from build123d import *

# Parameters (mm, degrees)
CUT_EXTRUDE1_DEPTH      = 10
CUT_EXTRUDE1_DEPTH_BACK = 10


with BuildPart() as part:
    # Sketch1 → Revolve1 (revolve)
    with BuildSketch(Plane(origin=(0, 0, 0), x_dir=(0, 0, -1), z_dir=(1, 0, 0))):
        Polygon((-25.1, 0), (-25.1, 5.717157288), (-24.817157288, 6), (205.333333333, 6), (205.333333333, 16), (216, 16), (216, 0), align=None)
    revolve(axis=Axis((0, 0, -216), (0, 0, 1)))

    # Sketch2 → Cut-Extrude1 (cut, two sides)
    with BuildSketch(Plane(origin=(0, 0, 0), x_dir=(1, 0, 0), z_dir=(0, 1, 0))) as cut_extrude1_sk:
        Polygon((-10, -39.1), (10, -39.1), (10, -19.1), (5, -19.1), (5, -31.1), (-5, -31.1), (-5, -19.1), (-10, -19.1), align=None)
    extrude(amount=CUT_EXTRUDE1_DEPTH, mode=Mode.SUBTRACT)
    extrude(cut_extrude1_sk.sketch, amount=-CUT_EXTRUDE1_DEPTH_BACK, mode=Mode.SUBTRACT)

    # Sketch3 → Revolve2 (revolve)
    with BuildSketch(Plane(origin=(0, 0, 0), x_dir=(0, 0, -1), z_dir=(1, 0, 0))):
        with BuildLine():
            Line((-47.1, 0), (-47.1, 4.233))
            Line((-47.1, 4.233), (-46.333, 5))
            Line((-46.333, 5), (-29.072729678, 5))
            Line((-29.072729678, 5), (-26.699415898, 4.136184428))
            ThreePointArc((-26.699415898, 4.136184428), (-26.598392718, 4.109115348), (-26.494203812, 4.1))
            Line((-26.494203812, 4.1), (-25.7, 4.1))
            ThreePointArc((-25.7, 4.1), (-25.275735931, 4.275735931), (-25.1, 4.7))
            Line((-25.1, 4.7), (-24.5, 4.7))
            Line((-24.5, 4.7), (-24.5, 0))
            Line((-24.5, 0), (-47.1, 0))
        make_face()
    revolve(axis=Axis((0, 0, 24.5), (0, 0, 1)))


solid = part.part
CAD build for the part. Positions are in the model's coordinates, mm. A direction names the side the tool comes from. Coordinates: 2 decimals unless noted, no trailing zeros. Order: outer loops, then holes, each group sorted by start corner. A loop starts at its lowest first (then second) coordinate and runs counter-clockwise, first axis right, second up.
Item 1: Band-saw the part on D-D on x = -10. List the corners of the cut face in (y, z), plus the area to 3 significant figures.
Check sheet entries:
outline: (-12.49, -216) - (12.49, -216) - (12.49, -205.33) - (-12.49, -205.33) - close
area: 266 mm2
Item 2: Drill centre lines: L1, parallel to Z at x = 3.5, y = 5.5; L2, parallel to X at y = 5, z = -145.5; L3, parallel to Y at x = 0.5, z = -32. Where is each one in solid material? Low to high.
Check sheet entries:
L1: z = -216 to -205.33
L2: x = -3.32 to 3.32
L3: y = -5.98 to 5.98
Item 3: 3-axis set-ups, long thin cutter, end or side, ignore diameter. For faces 1 (the face through (0, 0, -216)), 2 (the face through (4.88, -1.08, 37.58)), 3 (the face through (5, 0, 22)), 4 (the face through (-5, 0, 22)): which of +Z, -Z, +X, -X, +Y, -Y reach the whole face in a straight line?
Check sheet entries:
face 1: -Z, +X, -X, +Y, -Y
face 2: +Z
face 3: +Z, +X, +Y, -Y
face 4: +Z, -X, +Y, -Y
Item 4: Pin check, flat tips, straight feed: pin 1 Ø3 at (y, z) = (1, 22) entering from +X; pin 2 Ø4 at (x, y) = (12.5, -5) entering from +Z; pin 3 Ø5 at (y, z) = (-0.5, 21) entering from -X. Stop position of each tip, or through.
Check sheet entries:
pin 1: stops at x = 5
pin 2: stops at z = -205.33
pin 3: stops at x = -6
Item 5: Band-saw the part on C-C on z = 0. List the corners of the cut face in (x, y).
Check sheet entries:
outline: circle Ø12 at (0, 0)
Item 6: Band-saw the part on B-B on y = 0. List the corners of the cut face in (x, z), plus the area to 3 significant figures.
Check sheet entries:
outline: (-16, -216) - (16, -216) - (16, -205.33) - (6, -205.33) - (6, 19.1) - (5, 19.1) - (5, 25.1) - (4.7, 25.1) arc R0.6 cw to (4.1, 25.7) - (4.1, 26.49) arc R0.6 cw to (4.14, 26.7) - (5, 29.07) - (5, 46.33) - (4.23, 47.1) - (-4.23, 47.1) - (-5, 46.33) - (-5, 29.07) - (-4.14, 26.7) arc R0.6 cw to (-4.1, 26.49) - (-4.1, 25.7) arc R0.6 cw to (-4.7, 25.1) - (-5, 25.1) - (-5, 19.1) - (-6, 19.1) - (-6, -205.33) - (-16, -205.33) - close
area: 3,310 mm2
Item 7: Two-plate mould, pull along Z, no slides. Class faces 5 (the face through (0, -6, -92)), 6 (the face through (0, -7, -205.333)), 7 (the face through (-4.065, -0.534, 26.092)), 8 (the face through (4, -3, 25.1)): +Z half, -Z half, draft (parallel to the pull), parting line (faces both ways), or undercut.
Check sheet entries:
face 5: draft
face 6: +Z half
face 7: undercut
face 8: undercut
Item 8: Band-saw the part on A-A on x = 0. List the corners of the cut face in (y, z).
Check sheet entries:
outline: (-16, -216) - (16, -216) - (16, -205.33) - (6, -205.33) - (6, 24.82) - (5.72, 25.1) - (4.7, 25.1) arc R0.6 cw to (4.1, 25.7) - (4.1, 26.49) arc R0.6 cw to (4.14, 26.7) - (5, 29.07) - (5, 46.33) - (4.23, 47.1) - (-4.23, 47.1) - (-5, 46.33) - (-5, 29.07) - (-4.14, 26.7) arc R0.6 cw to (-4.1, 26.49) - (-4.1, 25.7) arc R0.6 cw to (-4.7, 25.1) - (-5.72, 25.1) - (-6, 24.82) - (-6, -205.33) - (-16, -205.33) - close
